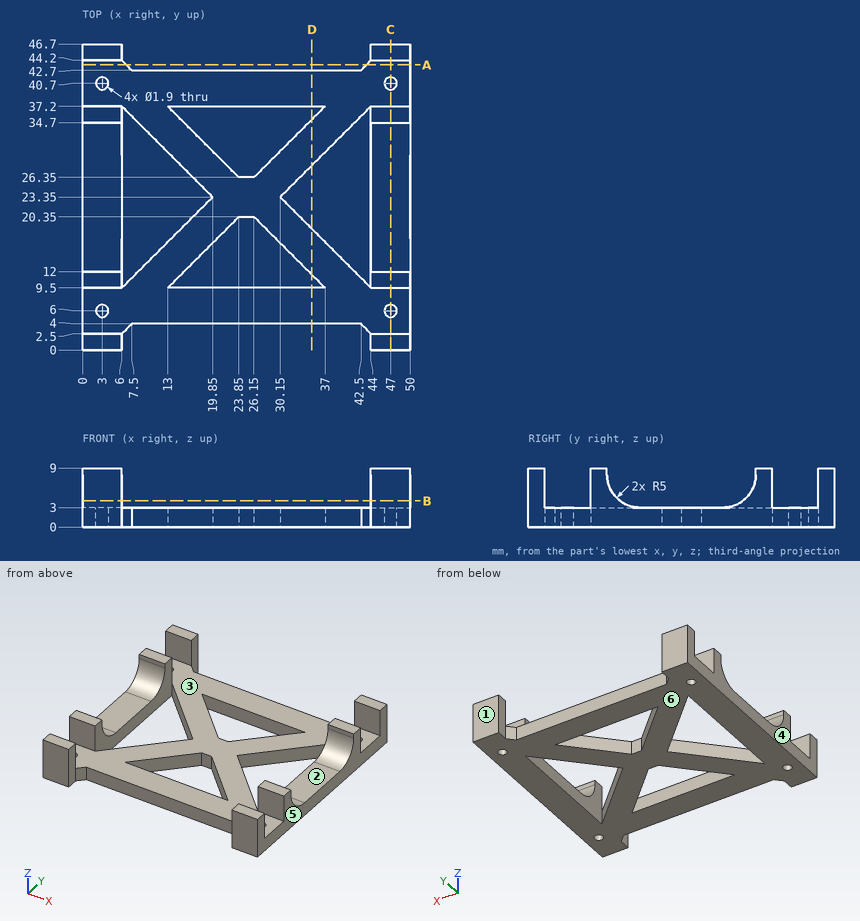
Answer from the drawing. Dimensions are ordinates in mm from the lowest x, y and z of the part. A direction names the side the tool comes from. Give positions to 0.01 mm unless a question says otherwise; leave off trailing zeros. Write each loop counter-clockwise with the first axis right and the second up, starting at its lowest first coordinate (ties: lowest second). Pieces come first, ordered by that corner, then holes. Notation, with made-up numbers: (11, 46.5) - (46, 46.5) arc R28 ccw to (46, 67.5) - close; hole circle Ø11 at (30.5, -22.5). An arc over 180 degrees is marked (long way). Answer in a Markdown table with one row per item. Add a question column.
Item 1: Section D-D, the plane x = 35 is taken. Write down the section's boundary in (y, z), and give its area (3 significant figures).
Item 2: Determine the mould class of the marked faces 3, 4, 5 and 6 for opening direction X: pulls with the +X half, pulls with the -X half, needs draft (parallel to the pull), parting line crosses it, or undercut.
Item 3: Find the intervals of material crossed by L1, parallel to X at y = 40.7, z = 1.6; L2, parallel to Y at x = 47, z = 2.2; L3, parallel to Y at x = 29, z = 1.5, in increasing order.
Item 4: Flat-ended cylindrical pins translate along their axes: P1, Ø2, axis at x = 14, y = 14.5, coming from the +Z side; P2, Ø0.7, axis at x = 24.5, z = 1.5, coming from the -Y side; P3, Ø3.5, axis at x = 25, z = 1.5, coming from the +Y side; P4, Ø3, axis at x = 3, y = 40.7, coming from the -Z side. Find the tip coordinate at first contact, or state that the pin passes through.
Item 5: Section B-B, the plane z = 4 is taken. Count the separate pieces of the cut face and the enclosed holes in it, and give its area (3 significant figures).
Item 6: Section C-C, the plane x = 47 is taken. Write down the section's boundary in (y, z), and give its area (3 significant figures).
Item 7: Section A-A, the plane y = 43.5 is taken. Write down the section's boundary in (x, z), and give its area (3 significant figures).
Item 8: A tool of negligible diameter and unlimited length cuts with its end or side. For the marked faces 1 and 2, from which of +Z, -Z, +X, -X, +Y, -Y can it reach the whole face along a straight path? Write none if from no direction.
Recorded:
| question | item | result |
|---|---|---|
| 1 | outline | (4, 0) - (9.5, 0) - (9.5, 3) - (4, 3) - close; (11.5, 0) - (18.5, 0) - (18.5, 3) - (11.5, 3) - close; (28.2, 0) - (35.2, 0) - (35.2, 3) - (28.2, 3) - close; (37.2, 0) - (42.7, 0) - (42.7, 3) - (37.2, 3) - close |
| 1 | area | 75.0 mm2 |
| 2 | face 3 | undercut |
| 2 | face 4 | pulls with the -X half |
| 2 | face 5 | pulls with the +X half |
| 2 | face 6 | needs draft |
| 3 | L1 | x = 0 to 2.05, 3.95 to 46.05, 47.95 to 50 |
| 3 | L2 | y = 0 to 5.05, 6.95 to 39.75, 41.65 to 46.7 |
| 3 | L3 | y = 4 to 9.5, 17.5 to 29.2, 37.2 to 42.7 |
| 4 | P1 | stops at z = 3 |
| 4 | P2 | stops at y = 4 |
| 4 | P3 | stops at y = 42.7 |
| 4 | P4 | stops at z = 0 |
| 5 | separate pieces | 8 |
| 5 | enclosed holes | 0 |
| 5 | area | 168 mm2 |
| 6 | outline | (0, 0) - (5.05, 0) - (5.05, 3) - (2.5, 3) - (2.5, 9) - (0, 9) - close; (6.95, 0) - (39.75, 0) - (39.75, 3) - (37.2, 3) - (37.2, 9) - (34.7, 9) - (34.7, 8) arc R5 cw to (29.7, 3) - (17, 3) arc R5 cw to (12, 8) - (12, 9) - (9.5, 9) - (9.5, 3) - (6.95, 3) - close; (41.65, 0) - (46.7, 0) - (46.7, 9) - (44.2, 9) - (44.2, 3) - (41.65, 3) - close |
| 6 | area | 199 mm2 |
| 7 | outline | (0, 0) - (6.7, 0) - (6.7, 3) - (0, 3) - close; (43.3, 0) - (50, 0) - (50, 3) - (43.3, 3) - close |
| 7 | area | 40.2 mm2 |
| 8 | face 1 | +Z, -Z, +X, -X, +Y |
| 8 | face 2 | +Z, +X, -X |
